Geometry: final body of the model. Coordinates: model frame, mm. A direction names the side the tool comes from. Give positions to 0.01 mm unless a question says otherwise; leave off trailing zeros. Order: outer loops, then holes, each group sorted by start corner. A loop starts at its lowest first (then second) coordinate and runs counter-clockwise, first axis right, second up. Notation, with made-up numbers: (33.25, 86.25) - (80.25, 86.25) arc R27 ccw to (80.25, 121.25) - close; hole circle Ø3 at (44.25, 36.5). An arc over 180 degrees is marked (long way). Put each result on its own line as item: value. Start each with the question number.
1. Section D-D on z = -16. Return the cut outline in (x, y), plus the area to 3 significant figures.
2. First-contact query: P1, Ø10, axis at y = -11.5, z = -15.5, coming from the +X side; P2, Ø1.6, axis at x = 7, z = -32.5, coming from the +Y side; P3, Ø3.5, axis at x = 33, y = 47.5, coming from the +Z side; P4, Ø3, axis at x = 9, z = -20, coming from the -Y side. Flat tips, straight axial feed; report the tip coordinate or a pass-through.
3. Section C-C on y = -8.5. Return the cut outline in (x, z).
4. Section A-A on z = -25. Return the cut outline in (x, y).
5. Mould query, pull axis Y, two halves, no side actions, for faces 1 (the flat face through (30, 42.25, -7)), 2 (the flat face through (12, -50, -10)), 3 (the cylindrical face through (43, -45, -9)), 4 (the flat face through (8, -14, -34)). Classes: pulls with the +Y half, pulls with the -Y half, needs draft (parallel to the pull), parting line crosses it, or undercut.
6. Ray query, line 1 along Y through (x, z) = (24, -8.5); line 2 along X through (y, z) = (-13.5, -9); line 3 along X through (y, z) = (43.5, -7). Return the intervals inside material, ascending. Write a range as from..to.
7. Section B-B on x = 30. Count the separate pieces of the cut face and the enclosed holes in it, plus the area to 4 significant figures.
8. Set-up query: faces 5 (the flat face through (7, 42.25, -30)), 6 (the flat face through (30, -18, -6)), 7 (the flat face through (26, -14, -8)). Return all of +Z, -Z, +X, -X, +Y, -Y with unobstructed straight access to the full face (end or side cutting, diameter ignored); none if empty.
from build123d import *

# Parameters (mm, degrees)
BOSS_EXTRUDE1_DEPTH      = 50
BOSS_EXTRUDE1_DEPTH_BACK = 50
BOSS_EXTRUDE2_DEPTH      = 50
BOSS_EXTRUDE2_DEPTH_BACK = 50
FILLET1_R                = 5
CUT_EXTRUDE2_DEPTH       = 40
CUT_EXTRUDE2_DEPTH_BACK  = 40
BOSS_EXTRUDE3_DEPTH      = 20
BOSS_EXTRUDE3_DEPTH_BACK = 20
CUT_EXTRUDE3_DEPTH       = 10
CUT_EXTRUDE3_DEPTH_BACK  = 10
SKETCH3_R                = 1.75
CUT_EXTRUDE1_DEPTH       = 118.038455219
SKETCH4_W                = 12.2
SKETCH4_H                = 5.5
CUT_EXTRUDE4_DEPTH       = 2
LPATTERN1_COUNT          = 4
LPATTERN1_PITCH          = 30
SKETCH6_W                = 12.2
SKETCH6_H                = 5.5
CUT_EXTRUDE5_DEPTH       = 2
LPATTERN2_COUNT          = 4
LPATTERN2_PITCH          = 30
SKETCH7_W                = 12.2
SKETCH7_H                = 4
CUT_EXTRUDE6_DEPTH       = 2
LPATTERN3_COUNT          = 4
LPATTERN3_PITCH          = 30
SKETCH8_W                = 12.2
SKETCH8_H                = 4
CUT_EXTRUDE7_DEPTH       = 2
LPATTERN4_COUNT          = 4
LPATTERN4_PITCH          = 30


with BuildPart() as part:
    # Sketch1 → Boss-Extrude1 (new, two sides: drawn at the far end of the back side and taken through both)
    with BuildSketch(Plane(origin=(0, 0, 0), x_dir=(1, 0, 0), z_dir=(0, 1, 0)).offset(-BOSS_EXTRUDE1_DEPTH_BACK)):
        Polygon((0, 0), (0, 20), (12, 20), (12, 12), (20, 12), (20, 0), align=None)
    extrude(amount=BOSS_EXTRUDE1_DEPTH + BOSS_EXTRUDE1_DEPTH_BACK)

    # Sketch2 → Boss-Extrude2 (add, two sides: drawn at the far end of the back side and taken through both)
    with BuildSketch(Plane(origin=(0, 0, 0), x_dir=(1, 0, 0), z_dir=(0, 1, 0)).offset(-BOSS_EXTRUDE2_DEPTH_BACK)):
        with BuildLine():
            Line((20, 12), (40, 12))
            ThreePointArc((40, 12), (43, 9), (40, 6))
            Line((40, 6), (20, 6))
            ThreePointArc((20, 6), (17, 9), (20, 12))
        make_face()
        with BuildLine():
            Line((12, 40), (12, 20))
            ThreePointArc((12, 20), (9, 17), (6, 20))
            Line((6, 20), (6, 40))
            ThreePointArc((6, 40), (9, 43), (12, 40))
        make_face()
    extrude(amount=BOSS_EXTRUDE2_DEPTH + BOSS_EXTRUDE2_DEPTH_BACK)

    # Fillet1
    fillet1_edges = [part.edges().sort_by_distance(p)[0] for p in [
        (0, 0, 0),
    ]]
    fillet(fillet1_edges, radius=FILLET1_R)

    # Sketch2_2 → Cut-Extrude2 (cut, two sides: drawn at the far end of the back side and taken through both)
    with BuildSketch(Plane(origin=(0, 0, 0), x_dir=(1, 0, 0), z_dir=(0, 1, 0)).offset(-CUT_EXTRUDE2_DEPTH_BACK)):
        with BuildLine():
            Line((20, 12), (40, 12))
            ThreePointArc((40, 12), (43, 9), (40, 6))
            Line((40, 6), (20, 6))
            ThreePointArc((20, 6), (17, 9), (20, 12))
        make_face()
        with BuildLine():
            Line((12, 40), (12, 20))
            ThreePointArc((12, 20), (9, 17), (6, 20))
            Line((6, 20), (6, 40))
            ThreePointArc((6, 40), (9, 43), (12, 40))
        make_face()
    extrude(amount=CUT_EXTRUDE2_DEPTH + CUT_EXTRUDE2_DEPTH_BACK, mode=Mode.SUBTRACT)

    # Sketch2_3 → Boss-Extrude3 (add, two sides: drawn at the far end of the back side and taken through both)
    with BuildSketch(Plane(origin=(0, 0, 0), x_dir=(1, 0, 0), z_dir=(0, 1, 0)).offset(-BOSS_EXTRUDE3_DEPTH_BACK)):
        with BuildLine():
            Line((20, 12), (40, 12))
            ThreePointArc((40, 12), (43, 9), (40, 6))
            Line((40, 6), (20, 6))
            ThreePointArc((20, 6), (17, 9), (20, 12))
        make_face()
        with BuildLine():
            Line((12, 40), (12, 20))
            ThreePointArc((12, 20), (9, 17), (6, 20))
            Line((6, 20), (6, 40))
            ThreePointArc((6, 40), (9, 43), (12, 40))
        make_face()
    extrude(amount=BOSS_EXTRUDE3_DEPTH + BOSS_EXTRUDE3_DEPTH_BACK)

    # Sketch2_4 → Cut-Extrude3 (cut, two sides: drawn at the far end of the back side and taken through both)
    with BuildSketch(Plane(origin=(0, 0, 0), x_dir=(1, 0, 0), z_dir=(0, 1, 0)).offset(-CUT_EXTRUDE3_DEPTH_BACK)):
        with BuildLine():
            Line((20, 12), (40, 12))
            ThreePointArc((40, 12), (43, 9), (40, 6))
            Line((40, 6), (20, 6))
            ThreePointArc((20, 6), (17, 9), (20, 12))
        make_face()
        with BuildLine():
            Line((12, 40), (12, 20))
            ThreePointArc((12, 20), (9, 17), (6, 20))
            Line((6, 20), (6, 40))
            ThreePointArc((6, 40), (9, 43), (12, 40))
        make_face()
    extrude(amount=CUT_EXTRUDE3_DEPTH + CUT_EXTRUDE3_DEPTH_BACK, mode=Mode.SUBTRACT)

    # Sketch3 → Cut-Extrude1 (cut, through all)
    with BuildSketch(Plane(origin=(0, 50, 0), x_dir=(1, 0, 0), z_dir=(0, 1, 0))):
        with Locations(Location((9, 40, 0), (0, 0, 270))):
            Circle(SKETCH3_R)
        with Locations(Location((9, 20, 0), (0, 0, 270))):
            Circle(SKETCH3_R)
        with Locations(Location((20, 9, 0), (0, 0, 270))):
            Circle(SKETCH3_R)
        with Locations(Location((40, 9, 0), (0, 0, 270))):
            Circle(SKETCH3_R)
        with Locations(Location((30, 9, 0), (0, 0, 270))):
            Circle(SKETCH3_R)
        with Locations(Location((9, 30, 0), (0, 0, 270))):
            Circle(SKETCH3_R)
    extrude(amount=-CUT_EXTRUDE1_DEPTH, mode=Mode.SUBTRACT)

    # Sketch4 → Cut-Extrude4 (cut)
    with BuildSketch(Plane.XY.offset(-6)):
        with Locations((30, 45)):
            Rectangle(SKETCH4_W, SKETCH4_H)
    cut_extrude4 = extrude(amount=-CUT_EXTRUDE4_DEPTH, mode=Mode.SUBTRACT)

    # LPattern1: Cut-Extrude4 ×4
    with Locations(*[(0, -i * LPATTERN1_PITCH, 0) for i in range(1, LPATTERN1_COUNT)]):
        add(cut_extrude4, mode=Mode.SUBTRACT)

    # Sketch6 → Cut-Extrude5 (cut)
    with BuildSketch(Plane.ZY.offset(-6)):
        with Locations((-30, 45)):
            Rectangle(SKETCH6_W, SKETCH6_H)
    cut_extrude5 = extrude(amount=-CUT_EXTRUDE5_DEPTH, mode=Mode.SUBTRACT)

    # LPattern2: Cut-Extrude5 ×4
    with Locations(*[(0, -i * LPATTERN2_PITCH, 0) for i in range(1, LPATTERN2_COUNT)]):
        add(cut_extrude5, mode=Mode.SUBTRACT)

    # Sketch7 → Cut-Extrude6 (cut)
    with BuildSketch(Plane.ZY.offset(-6)):
        with Locations((-30, 49.75)):
            Rectangle(SKETCH7_W, SKETCH7_H)
    cut_extrude6 = extrude(amount=-CUT_EXTRUDE6_DEPTH, mode=Mode.SUBTRACT)

    # LPattern3: Cut-Extrude6 ×4
    with Locations(*[(0, -i * LPATTERN3_PITCH, 0) for i in range(1, LPATTERN3_COUNT)]):
        add(cut_extrude6, mode=Mode.SUBTRACT)

    # Sketch8 → Cut-Extrude7 (cut)
    with BuildSketch(Plane.XY.offset(-6)):
        with Locations((30, 49.75)):
            Rectangle(SKETCH8_W, SKETCH8_H)
    cut_extrude7 = extrude(amount=-CUT_EXTRUDE7_DEPTH, mode=Mode.SUBTRACT)

    # LPattern4: Cut-Extrude7 ×4
    with Locations(*[(0, -i * LPATTERN4_PITCH, 0) for i in range(1, LPATTERN4_COUNT)]):
        add(cut_extrude7, mode=Mode.SUBTRACT)


solid = part.part
Resolved:
1. outline: (0, -50) - (12, -50) - (12, 50) - (0, 50) - close
1. area: 1,200 mm^2
2. P1: x = 42.6
2. P2: y = 42.25
2. P3: z = -8
2. P4: through
3. outline: (0, -20) - (6, -20) arc R3 cw to (12, -20) - (12, -12) - (20, -12) arc R3 cw to (20, -6) - (20, 0) - (5, 0) arc R5 ccw to (0, -5) - close
4. outline: (6, -50) - (12, -50) - (12, -40) - (8, -40) - (8, -47.75) - (6, -47.75) - close; (6, -20) - (12, -20) - (12, -10) - (8, -10) - (8, -17.75) - (6, -17.75) - close; (6, 10) - (12, 10) - (12, 20) - (8, 20) - (8, 12.25) - (6, 12.25) - close; (6, 40) - (12, 40) - (12, 50) - (8, 50) - (8, 42.25) - (6, 42.25) - close
5. face 1: pulls with the +Y half
5. face 2: pulls with the -Y half
5. face 3: needs draft
5. face 4: undercut
6. line 1: -50..-40, -20..-10, 10..20, 40..50
6. line 2: 0..18.25, 21.75..28.25, 31.75..38.25, 41.75..43
6. line 3: 0..23.9, 36.1..42.24
7. separate pieces: 8
7. enclosed holes: 0
7. area: 61.25 mm^2
8. face 5: -X, +Y
8. face 6: +Z, +X, +Y, -Y
8. face 7: +Z
